Read the model definition and answer for the solid it produces. Units are mm, in the model's axes. A direction names the side the tool comes from. Coordinates: 2 decimals unless noted, no trailing zeros. Loops run counter-clockwise (first coordinate to the right, second up) from the corner with the lowest first, then second, coordinate; pieces in that order, holes last.
Q1. Straight lines are drawn through the part: line 1 (X direction, y = -14.5, z = 51); line 2 (Z direction, x = 18, y = -15); line 3 (X direction, y = -6, z = 8.5). For each, find the intervals that lie inside material, in ascending order.
Q2. The mould has two halves that part along X. Classify faces 3 (the face through (27, -15, 6)), 4 (the face through (-21, 0, 36)), 5 (the face through (-26.9, -14.7, 54)): pulls with the +X half, pulls with the -X half, needs draft (parallel to the pull), parting line crosses it, or undercut.
Q3. Section D-D (y = -17.5) is taken. Give the vertices of the cut face in (x, z).
Q4. Section B-B (z = 4) is taken. Give the vertices of the cut face in (x, y).
Q5. Flat-ended cylindrical pins translate along their axes: P1, Ø3, axis at x = 24.5, z = 23, coming from the -Y side; P2, Ø3.5, axis at y = -0.5, z = 3.5, coming from the +X side; P3, Ø6, axis at y = 9.5, z = 19.5, coming from the +X side; P4, Ø1, axis at x = 24.5, z = 15.5, coming from the -Y side. Find the tip coordinate at first contact, or state that the pin passes through.
Q6. Section A-A (z = 40) is taken. Give the vertices of the cut face in (x, y).
Q7. Section C-C (x = 4) is taken. Give the vertices of the cut face in (y, z), then the cut area to 3 significant figures.
Q8. Which of the six approach directions +Z, -Z, +X, -X, +Y, -Y give full straight-line access (tool end or side, diameter ignored) to faces 1 (the face through (-27.1, 14.7, 54)), 2 (the face through (-20.844, 0, 33))?
Autodesk Fusion 360 part; units mm, degrees
sketch "Sketch1" plane through (0, 0, 0) normal (0, 0, 1) x (1, 0, 0)
  line L0 (33, 21) -> (-33, 21)
  line L1 (-33, 21) -> (-33, -21)
  line L2 (-33, -21) -> (33, -21)
  line L3 (33, -21) -> (33, 21)
  line L4 (33, 21) -> (-33, -21) construction
  line L5 (-33, 21) -> (33, -21) construction
  dimension "d1" = 66
  dimension "d2" = 42
extrude "Extrude1" add sketch "Sketch1" along normal blind 12
chamfer "Chamfer1" distance 12 angle 45 2 edges at (33, -21, 6) (33, 21, 6)
sketch "Sketch2" plane through (0, 0, 12) normal (0, 0, 1) x (-1, 0, 0)
  line L0 (-33, -9) -> (-21, -21)
  line L1 (-21, -21) -> (33, -21)
  line L2 (33, -21) -> (33, 21)
  line L3 (33, 21) -> (-21, 21)
  line L4 (-21, 21) -> (-33, 9)
  line L5 (-33, 9) -> (-33, -9)
  line L6 (33, -21) -> (21, -21)
  line L7 (21, -21) -> (21, 21)
  line L8 (21, 21) -> (33, 21)
  line L9 (33, 21) -> (33, -21)
  dimension "d6" = 12
extrude "Extrude2" add sketch "Sketch2" along normal blind 48 contours L1 L2 L3 L6 L7 L8 L9
fillet "Fillet1" radius 21 2 edges at (-27, -21, 60) (-27, 21, 60)
sketch "Sketch3" plane through (0, 0, 0) normal (0, 1, 0) x (1, 0, 0)
  line L0 (-20.8444, -53.9217) -> (-20.8444, -11.9217)
  line L1 (-20.8444, -11.9217) -> (33.1556, -11.9217)
  line L2 (33.1556, -11.9217) -> (-20.8444, -53.9217)
  dimension "d10" = 42
  dimension "d11" = 54
extrude "Extrude3" add sketch "Sketch3" along normal mid plane 12
equation "d7 = 60 mm - 12 mm"
equation "d11 = 66 mm - 12 mm"
Numbers:
1. line 1: x = -33 to -21
1. line 2: z = 0 to 12
1. line 3: x = -33 to 33
2. face 3: pulls with the +X half
2. face 4: undercut
2. face 5: needs draft
3. outline: (-33, 0) - (24.5, 0) - (24.5, 12) - (-21, 12) - (-21, 50.61) - (-33, 50.61) - close
4. outline: (-33, -21) - (21, -21) - (33, -9) - (33, 9) - (21, 21) - (-33, 21) - close
5. P1: passes through
5. P2: stops at x = 33
5. P3: stops at x = -21
5. P4: stops at y = -6
6. outline: (-33, -20.98) - (-21, -20.98) - (-21, 20.98) - (-33, 20.98) - close; (-20.84, -6) - (-2.95, -6) - (-2.95, 6) - (-20.84, 6) - close
7. outline: (-21, 0) - (21, 0) - (21, 12) - (6, 12) - (6, 34.6) - (-6, 34.6) - (-6, 12) - (-21, 12) - close
7. area: 775 mm2
8. face 1: +Z, +X, -X, +Y
8. face 2: +Z, +Y, -Y
